For this review, take the finished solid that the model builds, in its own axes (mm). Give positions to 0.01 mm unless a question says otherwise; leave off trailing zeros. Write each loop counter-clockwise with the first axis right and the second up, starting at its lowest first coordinate (ties: lowest second). Pieces come first, ordered by that corner, then holes.
1) Wall thickness on line 1 along Y through (x, z) = (0, 4); line 2 along Y through (x, z) = (20, 2.8); line 3 along X through (y, z) = (23, 3): over which ranges is each line inside the solid? List them lowest first.
2) We need section A-A on x = -20. Give the boundary of the cut face in (y, z), and give its area (3 significant figures).
3) For P1, Ø6, axis at x = 16.5, y = 19, coming from the +Z side; P2, Ø2, axis at y = -10.5, z = 0.5, coming from the +X side; P3, Ø1, axis at x = 18, z = 3.5, coming from the +Y side; P4, Ø1, axis at x = -4.5, z = 1, coming from the -Y side, all flat-tipped, find the tip position at first contact; note any pin that passes through.
4) We need section B-B on y = 0. Give the boundary of the cut face in (x, z), and give its area (3 significant figures).
5) We need section C-C on z = 2.9. Give the boundary of the cut face in (x, y).
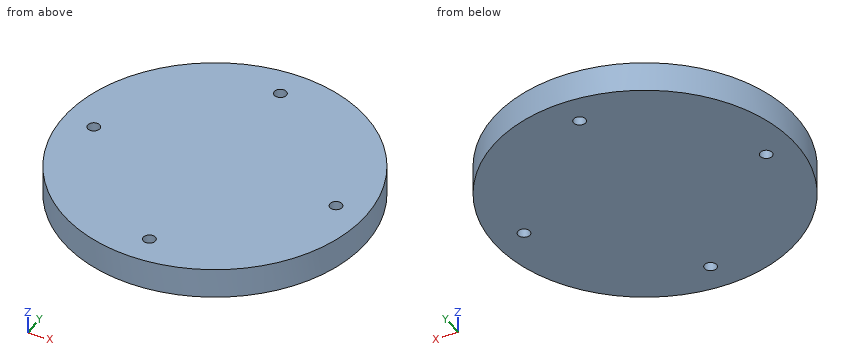
from build123d import *

# Parameters (mm, degrees)
F0_R     = 25
F1_DEPTH = 5
F2_R     = 1
F3_DEPTH = 5.001


with BuildPart() as f1:
    # F0 (on Top) → F1 (new body)
    with BuildSketch(Plane.XY):
        Circle(F0_R)
    extrude(amount=F1_DEPTH)

    # F2 (on face) → F3 (cut, through all)
    with BuildSketch(Plane.XY.offset(5)):
        with Locations((0, 20)):
            Circle(F2_R)
        with Locations((-20, 0)):
            Circle(F2_R)
        with Locations((0, -20)):
            Circle(F2_R)
        with Locations((20, 0)):
            Circle(F2_R)
    extrude(amount=-F3_DEPTH, mode=Mode.SUBTRACT)


solid = f1.part
Results list:
1. line 1: y = -25 to -21, -19 to 19, 21 to 25
1. line 2: y = -15 to -1, 1 to 15
1. line 3: x = -9.8 to 9.8
2. outline: (-15, 0) - (-1, 0) - (-1, 5) - (-15, 5) - close; (1, 0) - (15, 0) - (15, 5) - (1, 5) - close
2. area: 140 mm2
3. P1: stops at z = 5
3. P2: stops at x = 23.12
3. P3: stops at y = 17.85
3. P4: stops at y = -24.68
4. outline: (-25, 0) - (-21, 0) - (-21, 5) - (-25, 5) - close; (-19, 0) - (19, 0) - (19, 5) - (-19, 5) - close; (21, 0) - (25, 0) - (25, 5) - (21, 5) - close
4. area: 230 mm2
5. outline: circle Ø50 at (0, 0); hole circle Ø2 at (-20, 0); hole circle Ø2 at (0, -20); hole circle Ø2 at (0, 20); hole circle Ø2 at (20, 0)
